Part model, mm, in its own coordinate system. Round coordinates to 2 decimals unless told otherwise and drop trailing zeros. Write each loop counter-clockwise with the first axis right and the second up, starting at its lowest first coordinate (ties: lowest second). Pieces come first, ordered by that corner, then holes.
```python
from build123d import *

# Parameters (mm, degrees)
SKETCH1_R           = 41.656
BOSS_EXTRUDE1_DEPTH = 38.1
SKETCH2_R           = 3.18135
CUT_EXTRUDE1_DEPTH  = 29.464
CIRPATTERN1_COUNT   = 6
SKETCH3_R           = 46.1518
SKETCH3_R_2         = 41.656
BOSS_EXTRUDE2_DEPTH = 57.15
FILLET1_R           = 12.7


with BuildPart() as part:
    # Sketch1 → Boss-Extrude1 (new body)
    with BuildSketch(Plane(origin=(0, 0, 0), x_dir=(1, 0, 0), z_dir=(0, 1, 0))):
        Polygon((0, -60.565197939), (52.451, -30.282598969), (52.451, 30.282598969), (0, 60.565197939), (-52.451, 30.282598969), (-52.451, -30.282598969), align=None)
        with Locations(Location((0, 0, 0), (0, 0, 90))):
            Circle(SKETCH1_R, mode=Mode.SUBTRACT)
    extrude(amount=BOSS_EXTRUDE1_DEPTH)

    # Sketch2 → Cut-Extrude1 (cut)
    with BuildSketch(Plane.ZY.offset(52.451)):
        with Locations((0, 19.05)):
            Circle(SKETCH2_R)
    cut_extrude1 = extrude(amount=-CUT_EXTRUDE1_DEPTH, mode=Mode.SUBTRACT)

    # CirPattern1: Cut-Extrude1 ×6 about axis
    cirpattern1_axis = Axis((0, 38.1, 0), (0, 1, 0))
    for i in range(1, CIRPATTERN1_COUNT):
        add(cut_extrude1.rotate(cirpattern1_axis, i * 360 / CIRPATTERN1_COUNT), mode=Mode.SUBTRACT)

    # Sketch3 → Boss-Extrude2 (add)
    with BuildSketch(Plane(origin=(-52.451, 38.1, -30.282598969), x_dir=(1, 0, 0), z_dir=(0, -1, 0))):
        with Locations(Location((52.451, 30.282598969, 0), (0, 0, 270))):
            Circle(SKETCH3_R)
        with Locations(Location((52.451, 30.282598969, 0), (0, 0, 270))):
            Circle(SKETCH3_R_2, mode=Mode.SUBTRACT)
    extrude(amount=-BOSS_EXTRUDE2_DEPTH)

    # Fillet1
    fillet1_edges = [part.edges().sort_by_distance(p)[0] for p in [
        (-52.451, 19.05, 30.282598969),
        (-52.451, 19.05, -30.282598969),
        (0, 19.05, -60.565197939),
        (52.451, 19.05, -30.282598969),
        (52.451, 19.05, 30.282598969),
        (0, 19.05, 60.565197939),
    ]]
    fillet(fillet1_edges, radius=FILLET1_R)


solid = part.part
```
Q1. Drop flat-ended pins along their axis: pin 1 (1 mm diameter, centred on y = 83, z = -35, fed in from -X); pin 2 (5 mm diameter, centred on y = 54, z = -34, fed in from +X); pin 3 (2 mm diameter, centred on x = 3, y = 63, fed in from -Z); pin 4 (4 mm diameter, centred on y = 19.05, z = 0, fed in from +X). Give the stop position or say it passes through.
Values follow:
pin 1: stops at x = -30.66
pin 2: stops at x = 33.73
pin 3: stops at z = -46.11
pin 4: passes through
Q2. Cut at A-A on z = 0. Write the cut outline in (x, y).
Values follow:
outline: (-52.45, 0) - (-41.66, 0) - (-41.66, 15.87) - (-52.45, 15.87) - close; (-52.45, 22.23) - (-41.66, 22.23) - (-41.66, 95.25) - (-46.15, 95.25) - (-46.15, 38.1) - (-52.45, 38.1) - close; (41.66, 0) - (52.45, 0) - (52.45, 15.87) - (41.66, 15.87) - close; (41.66, 22.23) - (52.45, 22.23) - (52.45, 38.1) - (46.15, 38.1) - (46.15, 95.25) - (41.66, 95.25) - close
Q3. Cut at B-B on x = 0. Write the cut outline in (y, z), plus the area to 3 significant figures.
Values follow:
outline: (0, -58.6) - (38.1, -58.6) - (38.1, -46.15) - (95.25, -46.15) - (95.25, -41.66) - (0, -41.66) - close; (0, 41.66) - (95.25, 41.66) - (95.25, 46.15) - (38.1, 46.15) - (38.1, 58.6) - (0, 58.6) - close
area: 1,810 mm2
Q4. Cut at D-D on x = 43.5. Write the cut outline in (y, z), plus the area to 3 significant figures.
Values follow:
outline: (0, -35.45) - (38.1, -35.45) - (38.1, -15.42) - (95.25, -15.42) - (95.25, 15.42) - (38.1, 15.42) - (38.1, 35.45) - (0, 35.45) - close; hole circle Ø6.36 at (19.05, 0)
area: 4,430 mm2
Q5. Wall check: L1, parallel to Y at x = -45.25, z = 0; L2, parallel to Y at x = -48, z = 0; L3, parallel to Z at x = -12.5, y = 8. Give the ranges that are in metal, low to high.
Values follow:
L1: y = 0 to 15.87, 22.23 to 95.25
L2: y = 0 to 15.87, 22.23 to 38.1
L3: z = -53.35 to -39.74, 39.74 to 53.35
Q6. Mould opens along Z. For faces 1 (the cylindrical face through (22.937, 15.944, 41.108)), 2 (the cylindrical face through (-50.796, 19.317, -29.219)), 3 (the flat face through (-43, 38.1, -18)), 4 (the cylindrical face through (2.029, 66.275, 46.107)) say: +Z half, -Z half, draft (parallel to the pull), parting line (faces both ways), or undercut.
Values follow:
face 1: undercut
face 2: -Z half
face 3: draft
face 4: parting line
Q7. Cut at C-C on y = 29.5. Write the cut outline in (x, z), plus the area to 3 significant figures.
Values follow:
outline: (-52.45, -22.95) arc R12.7 ccw to (-46.1, -33.95) - (-6.35, -56.9) arc R12.7 ccw to (6.35, -56.9) - (46.1, -33.95) arc R12.7 ccw to (52.45, -22.95) - (52.45, 22.95) arc R12.7 ccw to (46.1, 33.95) - (6.35, 56.9) arc R12.7 ccw to (-6.35, 56.9) - (-46.1, 33.95) arc R12.7 ccw to (-52.45, 22.95) - close; hole circle Ø83.31 at (0, 0)
area: 4,030 mm2
